Autodesk Inventor part; units mm, degrees
ref_plane "YZ Plane" through (0, 0, 0) normal (1, 0, 0) x (0, 1, 0)
ref_plane "XZ Plane" through (0, 0, 0) normal (0, 1, 0) x (-1, 0, 0)
ref_plane "XY Plane" through (0, 0, 0) normal (0, 0, 1) x (1, 0, 0)
sketch "스케치1" plane through (0, 0, 0) normal (1, 0, 0) x (0, 1, 0)
  line L0 (0, 0) -> (0, 30)
  line L1 (0, 0) -> (30, 0) construction
  line L2 (0, 30) -> (0, 50)
  line L3 (0, 50) -> (31.958, 50)
  line L4 (0, 0) -> (17.3205, 30)
  line L5 (0, 0) -> (34.641, 0) construction
  line L6 (17.3205, 30) -> (32.724, 48.3572)
  arc A0 (32.724, 48.3572) -> (31.958, 50) centre (31.958, 49) ccw
  point P0 (34.1025, 50)
  dimension "d0" = 30
  dimension "d1" = 90
  dimension "d2" = 20
  dimension "d3" = 60
  dimension "d4" = 170
  dimension "d7" = 1
extrude "돌출1" add sketch "스케치1" along normal blind 5
properties part number "앞판바깥막이" material "알루미늄 6061"
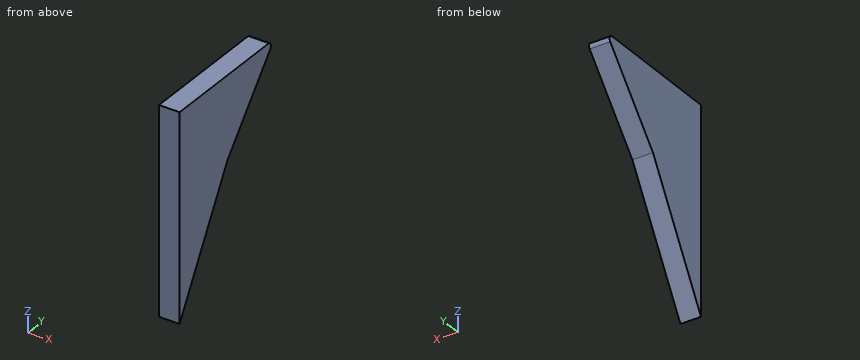
The model under review builds one solid part; all positions refer to its coordinate system, in mm. Give positions to 0.01 mm unless a question says otherwise; leave off trailing zeros. Write each loop counter-clockwise with the first axis right and the second up, starting at its lowest first coordinate (ties: lowest second). Pieces come first, ordered by that corner, then holes.
1. Wall thickness on L1, parallel to Z at x = 4.4, y = 25; L2, parallel to Y at x = 1.75, z = 27.5; L3, parallel to Y at x = 0.5, z = 43: over which ranges is each line inside the solid? List them lowest first.
2. Add section B-B, the plane y = 15. Write out the cut boundary in (x, z).
3. Add section C-C, the plane z = 25.5. Write out the cut boundary in (x, y), plus the area to 3 significant figures.
4. For P1, Ø1, axis at x = 1, z = 44.5, coming from the +Y side, flat-tipped, find the tip position at first contact; note if it passes through.
5. Add section A-A, the plane x = 2.6. Write out the cut boundary in (y, z).
Worked answers:
1. L1: z = 39.15 to 50
1. L2: y = 0 to 15.88
1. L3: y = 0 to 28.23
2. outline: (0, 25.98) - (5, 25.98) - (5, 50) - (0, 50) - close
3. outline: (0, 0) - (5, 0) - (5, 14.72) - (0, 14.72) - close
3. area: 73.6 mm2
4. P1: stops at y = 29.91
5. outline: (0, 0) - (17.32, 30) - (32.72, 48.36) arc R1 ccw to (31.96, 50) - (0, 50) - close
